Here's how the part is built. I have some questions about the finished solid (model axes, mm). Face numbers are marked on the shaded views. Give positions to 0.01 mm unless a question says otherwise; leave off trailing zeros. Loops run counter-clockwise (first coordinate to the right, second up) from the corner with the lowest first, then second, coordinate; pieces in that order, holes last. Notation, with made-up numbers: M -13.75,84 L 42.25,84 A22 cw 42.25,98 Z; hole C 16,30.5 d11. An arc over 180 degrees is marked long. Write item = value, one per line. Start each with the question number.
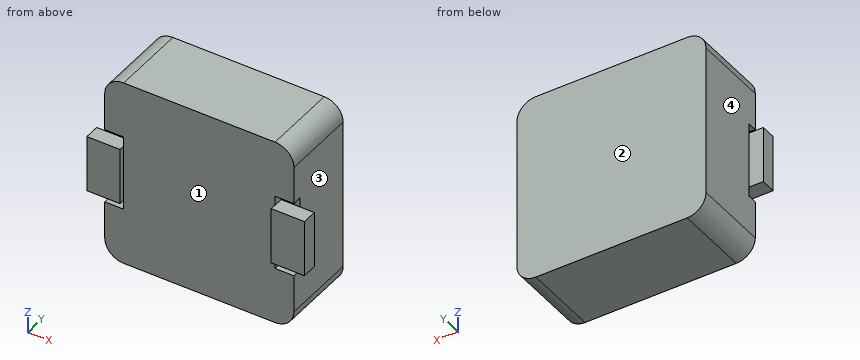
```python
from build123d import *

# Parameters (mm, degrees)
BOSS_EXTRUDE1_DEPTH = 4
SKETCH2_W           = 2
SKETCH2_H           = 4
CUT_EXTRUDE1_DEPTH  = 0.5
SKETCH3_W           = 1.75
SKETCH3_H           = 3
SKETCH3_W_2         = 1.75632414
BOSS_EXTRUDE2_DEPTH = 0.8


with BuildPart() as part:
    # Sketch1 → Boss-Extrude1 (new body)
    with BuildSketch(Plane(origin=(0, 0, 0), x_dir=(1, 0, 0), z_dir=(0, 1, 0))):
        with BuildLine():
            Line((-4, -5), (4, -5))
            ThreePointArc((4, -5), (4.707106781, -4.707106781), (5, -4))
            Line((5, -4), (5, 4))
            ThreePointArc((5, 4), (4.707106781, 4.707106781), (4, 5))
            Line((4, 5), (-4, 5))
            ThreePointArc((-4, 5), (-4.707106781, 4.707106781), (-5, 4))
            Line((-5, 4), (-5, -4))
            ThreePointArc((-5, -4), (-4.707106781, -4.707106781), (-4, -5))
        make_face()
    extrude(amount=BOSS_EXTRUDE1_DEPTH)

    # Sketch2 → Cut-Extrude1 (cut)
    with BuildSketch(Plane(origin=(0, 0, 0), x_dir=(1, 0, 0), z_dir=(0, 1, 0))):
        with Locations((-5, 0)):
            Rectangle(SKETCH2_W, SKETCH2_H)
        with Locations((5, 0)):
            Rectangle(SKETCH2_W, SKETCH2_H)
    extrude(amount=CUT_EXTRUDE1_DEPTH, mode=Mode.SUBTRACT)

    # Sketch3 → Boss-Extrude2 (add)
    with BuildSketch(Plane.XZ.offset(-0.5)):
        with Locations((-4.875, 0)):
            Rectangle(SKETCH3_W, SKETCH3_H)
        with Locations((4.87183793, 0)):
            Rectangle(SKETCH3_W_2, SKETCH3_H)
    extrude(amount=BOSS_EXTRUDE2_DEPTH)


solid = part.part
```
Q1. If I drill on line 1 along X through (y, z) = (0.1, 2.5); line 2 along Y through (x, z) = (2, -3); line 3 along X through (y, z) = (2, 4.75), over which ranges is the centre line in solid material (lowest first)?
Q2. If we section it at D-D, the plane x = 3.5: List the corners of the cut face in (y, z) for me.
Q3. Will these pins go through, and if not, where does the flat tip stop? pin 1 (0.6 mm diameter, centred on x = 4.5, z = 2, fed in from -Y); pin 2 (0.6 mm diameter, centred on x = -4.5, y = 0, fed in from -Z); pin 3 (1.2 mm diameter, centred on y = 1.5, z = 1, fed in from -X).
Q4. If we section it at A-A, the plane y = 2.1: List the corners of the cut face in (x, z) for me.
Q5. If we section it at B-B, the plane x = -4.25: List the corners of the cut face in (y, z) for me.
Q6. If we section it at C-C, the plane z = -2.25: List the corners of the cut face in (x, y) for me.
Q7. We'd pull the mould along X, two halves only. Please class the marked faces 1, 2, 3 and 4: pulls with the +X half, pulls with the -X half, needs draft (parallel to the pull), parting line crosses it, or undercut.
Resolved:
q1.line_1 = -5 to 5
q1.line_2 = 0 to 4
q1.line_3 = -4.66 to 4.66
q2.outline = M 0,-5 L 4,-5 L 4,5 L 0,5 Z
q3.pin_1 = 0
q3.pin_2 = -4.98
q3.pin_3 = -5
q4.outline = M -5,-4 A1 ccw -4,-5 L 4,-5 A1 ccw 5,-4 L 5,4 A1 ccw 4,5 L -4,5 A1 ccw -5,4 Z
q5.outline = M -0.3,-1.5 L 0.5,-1.5 L 0.5,-2 L 0,-2 L 0,-4.97 L 4,-4.97 L 4,4.97 L 0,4.97 L 0,2 L 0.5,2 L 0.5,1.5 L -0.3,1.5 Z
q6.outline = M -5,0 L 5,0 L 5,4 L -5,4 Z
q7.face_1 = undercut
q7.face_2 = needs draft
q7.face_3 = pulls with the +X half
q7.face_4 = pulls with the -X half
